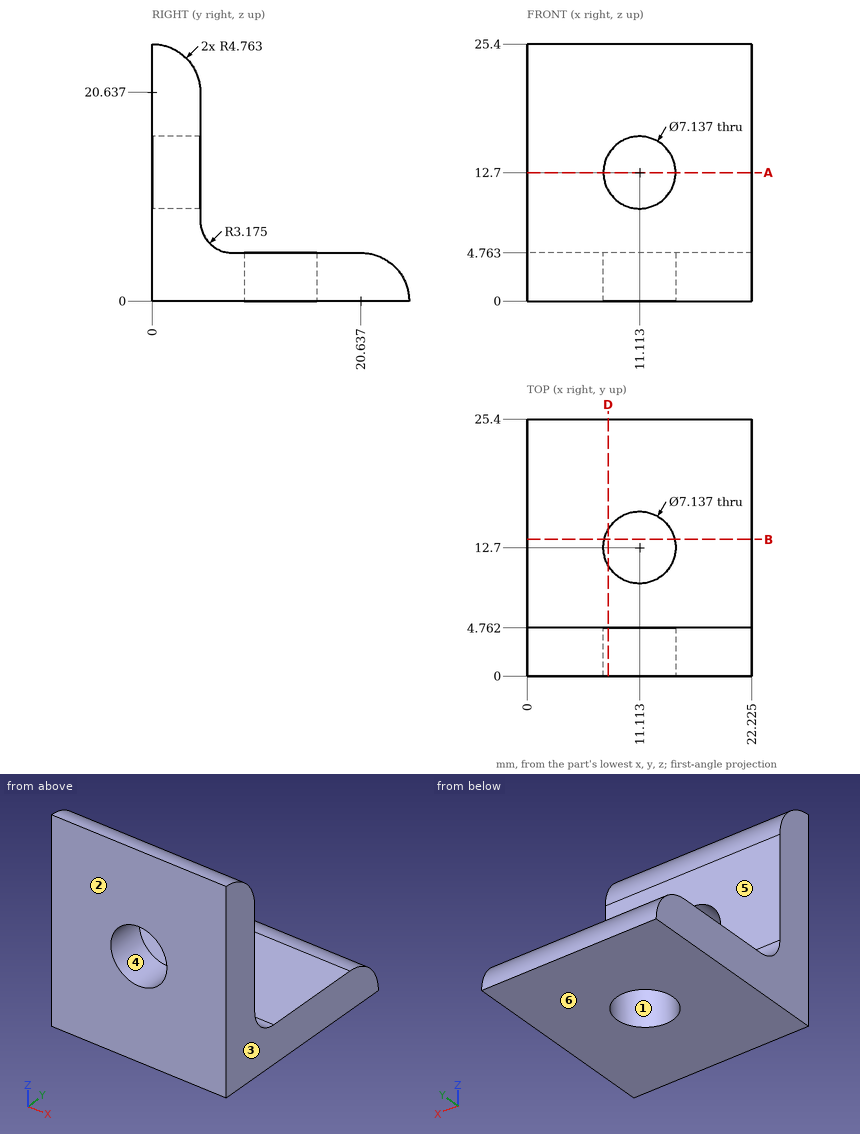
Check sheet for the drawn part. Datum: minimum x, y, z corner. Units: mm. A direction names the side the tool comes from. Round coordinates to 2 decimals unless told otherwise and drop trailing zeros. Write each loop counter-clockwise with the first axis right and the second up, starting at its lowest first coordinate (ties: lowest second). Pieces come first, ordered by that corner, then holes. Notation, with made-up numbers: (-16, -16) -> (37, -16) arc R8 cw to (37, -1) -> close; hole circle Ø5 at (39.5, 58). An arc over 180 degrees is marked (long way). One line per item, written item: value. Start each with the question number.
(1) Cross-section at D-D, the plane x = 8. Give the number of separate pieces and of enclosed holes in the cut face.
(2) Scan lines: line 1 (X direction, y = 2.35, z = 12.7) (1 decimal); line 2 (Y direction, x = 18.5, z = 20). Record each from-to range of solid material in increasing order. Write a range as [from, to].
(3) Draft check along X on the marked faces 1, 2, 3 and 4. Enter one of: +X half, -X half, draft (parallel to the pull), parting line (faces both ways), or undercut.
(4) Cross-section at B-B, the plane y = 13.5. Record the cut outline in (x, z) (1 decimal).
(5) Cross-section at A-A, the plane z = 12.7. Record the cut outline in (x, y) (1 decimal).
(6) Access from +Z, -Z, +X, -X, +Y, -Y to the whole of each face (thin tool, end or side, straight path). Record for the marked faces 5 and 6.
(7) Go/stop test with flat-tipped pins: pin 1 Ø1.5 at (x, z) = (18.5, 22) entering from +Y; pin 2 Ø1.5 at (x, z) = (5, 14) entering from +Y; pin 3 Ø11.5 at (x, z) = (11.11, 12.7) entering from +Y. Record where each tip stops, or that it passes through.
Answer:
1. separate pieces: 3
1. enclosed holes: 0
2. line 1: [0, 7.5], [14.7, 22.2]
2. line 2: [0, 4.76]
3. face 1: undercut
3. face 2: draft
3. face 3: +X half
3. face 4: undercut
4. outline: (0, 0) -> (7.6, 0) -> (7.6, 4.8) -> (0, 4.8) -> close; (14.6, 0) -> (22.2, 0) -> (22.2, 4.8) -> (14.6, 4.8) -> close
5. outline: (0, 0) -> (7.5, 0) -> (7.5, 4.8) -> (0, 4.8) -> close; (14.7, 0) -> (22.2, 0) -> (22.2, 4.8) -> (14.7, 4.8) -> close
6. face 5: +Z, +X, -X, +Y
6. face 6: -Z, +X, -X, +Y, -Y
7. pin 1: y = 4.72
7. pin 2: y = 4.76
7. pin 3: y = 4.92
